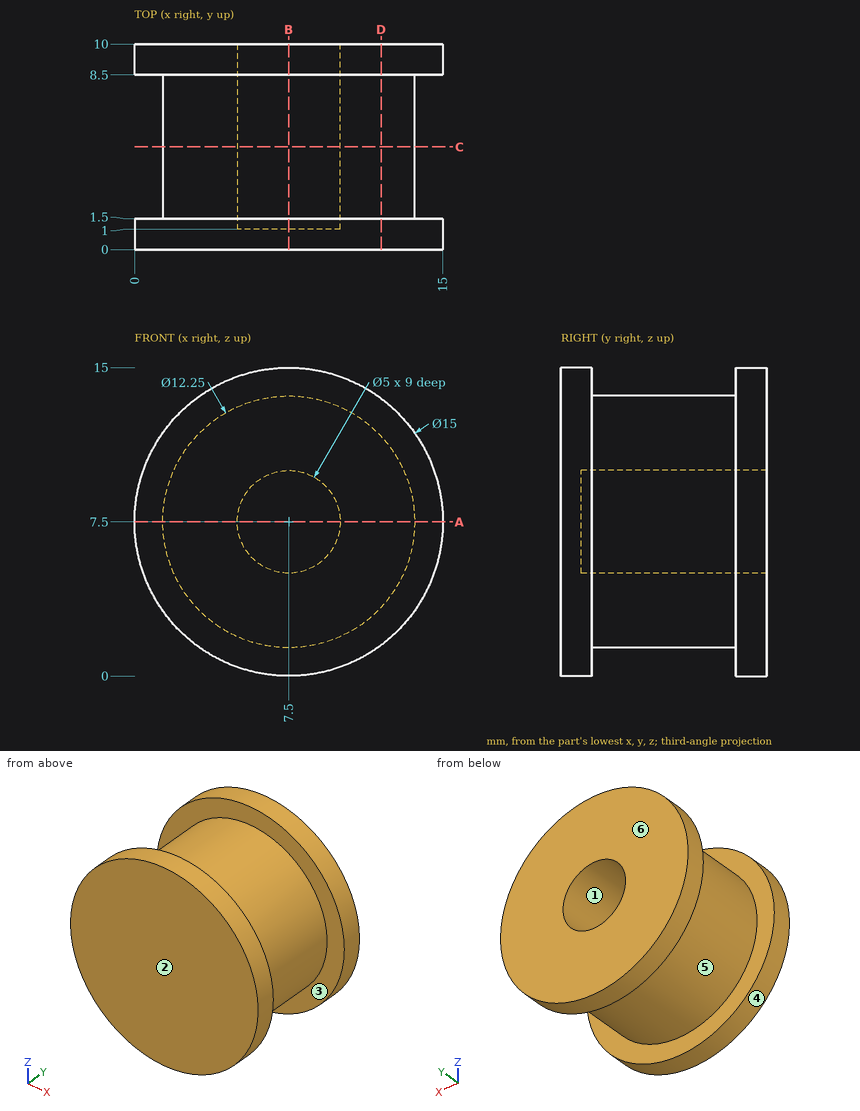
The figure shows three views and two pictorial views of one solid part (mm, origin at its lowest corner). Answer the questions. A direction names the side the tool comes from. Coordinates: 2 decimals unless noted, no trailing zeros. Loops run counter-clockwise (first coordinate to the right, second up) from the corner with the lowest first, then second, coordinate; pieces in that order, holes last. Notation, with made-up numbers: (53, -16.75) - (100, -16.75) arc R25 cw to (100, 12.25) - close; hole circle Ø5 at (33.25, 46). An arc over 180 degrees is marked (long way). Write item = value, one per line.
1) Section D-D (x = 12) is taken. Determine the outline of the cut face in (y, z).
Responses:
outline = (0, 1.5) - (1.5, 1.5) - (1.5, 3.34) - (8.5, 3.34) - (8.5, 1.5) - (10, 1.5) - (10, 13.5) - (8.5, 13.5) - (8.5, 11.66) - (1.5, 11.66) - (1.5, 13.5) - (0, 13.5) - close
2) Determine the mould class of the marked faces 4, 5 and 6 for opening direction Y: pulls with the +Y half, pulls with the -Y half, needs draft (parallel to the pull), parting line crosses it, or undercut.
Responses:
face_4 = needs draft
face_5 = undercut
face_6 = pulls with the +Y half
3) Each of these flat-tipped pins is pushed along its axis until it touches: P1, Ø1.5, axis at x = 4.5, y = 2, coming from the -Z side; P2, Ø1, axis at x = 12, y = 4.5, coming from the -Z side. Where does it stop, or does it pass through?
Responses:
P1 = 0.41
P2 = 2.86
4) Find the intervals of material crossed by line 1 along Z through (x, y) = (7.5, 4) (3 decimals); line 2 along Y through (x, z) = (1.25, 11), in increasing order.
Responses:
line_1 = 1.375 to 5, 10 to 13.625
line_2 = 0 to 1.5, 8.5 to 10
5) Which of the six approach directions +Z, -Z, +X, -X, +Y, -Y give full straight-line access (tool end or side, diameter ignored) to the marked faces 1, 2 and 3?
Responses:
face_1 = +Y
face_2 = +Z, -Z, +X, -X, -Y
face_3 = none
6) Section C-C (y = 5) is taken. Determine the outline of the cut face in (x, z) (3 decimals), plus the area to 3 significant figures.
Responses:
outline = circle Ø12.25 at (7.5, 7.5); hole circle Ø5 at (7.5, 7.5)
area = 98.2 mm^2
7) Section B-B (x = 7.5) is taken. Determine the outline of the cut face in (y, z) (3 decimals).
Responses:
outline = (0, 0) - (1.5, 0) - (1.5, 1.375) - (8.5, 1.375) - (8.5, 0) - (10, 0) - (10, 5) - (1, 5) - (1, 10) - (10, 10) - (10, 15) - (8.5, 15) - (8.5, 13.625) - (1.5, 13.625) - (1.5, 15) - (0, 15) - close
8) Section A-A (z = 7.5) is taken. Determine the outline of the cut face in (x, y) (3 decimals).
Responses:
outline = (0, 0) - (15, 0) - (15, 1.5) - (13.625, 1.5) - (13.625, 8.5) - (15, 8.5) - (15, 10) - (10, 10) - (10, 1) - (5, 1) - (5, 10) - (0, 10) - (0, 8.5) - (1.375, 8.5) - (1.375, 1.5) - (0, 1.5) - close
